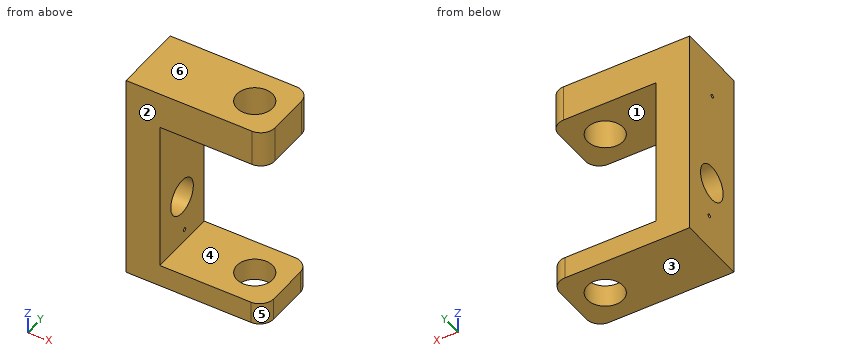
```python
from build123d import *

# Parameters (mm, degrees)
F0_W      = 50.8
F0_H      = 25.4
F1_DEPTH  = 76.2
F2_W      = 38.502306
F2_H      = 62.993251
F3_DEPTH  = 50.8
F5_R      = 6.477
F6_DEPTH  = 25.4
F7_W      = 25.4
F7_H      = 8.050508
F8_DEPTH  = 38.1
F4_R      = 6.477
F9_DEPTH  = 101.6
F10_R     = 5.08
F11_R     = 0.652616
F12_DEPTH = 25.4


with BuildPart() as f1:
    # F0 (on Top) → F1 (new body)
    with BuildSketch(Plane.XY):
        with Locations((-25.4, 12.7)):
            Rectangle(F0_W, F0_H)
    extrude(amount=F1_DEPTH)

    # F2 (on face) → F3 (cut)
    with BuildSketch(Plane.XZ):
        with Locations((-19.251153, 31.496625)):
            Rectangle(F2_W, F2_H)
    extrude(amount=-F3_DEPTH, mode=Mode.SUBTRACT)

    # F5 (on face) → F6 (cut)
    with BuildSketch(Plane(origin=(-50.8, 0, 0), x_dir=(0, -1, 0), z_dir=(-1, 0, 0))):
        with Locations((-12.7, 26.55393)):
            Circle(F5_R)
    extrude(amount=-F6_DEPTH, mode=Mode.SUBTRACT)

    # F7 (on face) → F8 (join)
    with BuildSketch(Plane.YZ.offset(-38.502306)):
        with Locations((12.7, 4.025254)):
            Rectangle(F7_W, F7_H)
    extrude(amount=F8_DEPTH)

    # F4 (on face) → F9 (cut)
    with BuildSketch(Plane.XY.offset(76.2)):
        with Locations((-12.11443, 12.7)):
            Circle(F4_R)
    extrude(amount=-F9_DEPTH, mode=Mode.SUBTRACT)

    # F10
    f10_edges = [f1.edges().sort_by_distance(p)[0] for p in [
        (0, 0, 69.596625),
        (-0.402306, 0, 4.025254),
        (-0.402306, 25.4, 4.025254),
        (0, 25.4, 69.596625),
    ]]
    fillet(f10_edges, radius=F10_R)

    # F11 (on face) → F12 (cut)
    with BuildSketch(Plane(origin=(-50.8, 0, 0), x_dir=(0, -1, 0), z_dir=(-1, 0, 0))):
        with Locations((-12.464834, 61.265279)):
            Circle(F11_R)
        with Locations((-14.175368, 12.515864)):
            Circle(F11_R)
    extrude(amount=-F12_DEPTH, mode=Mode.SUBTRACT)


solid = f1.part
```
Geometry check sheet. Reference: the model listing, model coordinates, mm. Face numbers are marked on the shaded views. A direction names the side the tool comes from. Give positions to 0.01 mm unless a question says otherwise; leave off trailing zeros. Loops run counter-clockwise (first coordinate to the right, second up) from the corner with the lowest first, then second, coordinate; pieces in that order, holes last. Notation, with made-up numbers: M -19.75,77 L 4.25,77 A15 cw 4.25,91 Z; hole C 20.25,-38 d5. An arc over 180 degrees is marked long. Write item = value, one per line.
(1) Sectioned sample at D-D, the plane z = 6.5. Record the cut outline in (x, y).
Answer below:
outline = M -50.8,0 L -5.48,0 A5.08 ccw -0.4,5.08 L -0.4,20.32 A5.08 ccw -5.48,25.4 L -50.8,25.4 Z; hole C -12.11,12.7 d12.95
(2) Release check for a two-part mould opening along Z. For the marked faces 3, 4, 5 and 6 record: released by +Z, released by -Z, zero draft, split by the parting line, or undercut.
Answer below:
face_3 = released by -Z
face_4 = undercut
face_5 = zero draft
face_6 = released by +Z
(3) Sectioned sample at C-C, the plane y = 10.5. Record the cut outline in (x, z).
Answer below:
outline = M -50.8,0 L -18.21,0 L -18.21,8.05 L -38.5,8.05 L -38.5,20.46 L -50.8,20.46 Z; M -50.8,32.65 L -38.5,32.65 L -38.5,62.99 L -18.21,62.99 L -18.21,76.2 L -50.8,76.2 Z; M -6.02,0 L -0.4,0 L -0.4,8.05 L -6.02,8.05 Z; M -6.02,62.99 L 0,62.99 L 0,76.2 L -6.02,76.2 Z
(4) Gauge pin test, flat ends, axial feed: pin 1 Ø10 at (y, z) = (17, 23.5) entering from +X; pin 2 Ø4 at (y, z) = (11.5, 3.5) entering from +X. Record the tip position at first contact, or that the pin passes through.
Answer below:
pin_1 = -38.5
pin_2 = -0.4
(5) Tool access check on the marked faces 1 and 2. Record the directions out of +Z, -Z, +X, -X, +Y, -Y that give a thin tool (end or side, any length) a straight path to the whole face; none if there is none.
Answer below:
face_1 = +X, +Y, -Y
face_2 = +Z, -Z, +X, -X, -Y
(6) Sectioned sample at A-A, the plane x = -28.5. Record the cut outline in (y, z).
Answer below:
outline = M 0,0 L 25.4,0 L 25.4,8.05 L 0,8.05 Z; M 0,62.99 L 25.4,62.99 L 25.4,76.2 L 0,76.2 Z
(7) Sectioned sample at B-B, the plane z = 70.5. Record the cut outline in (x, y).
Answer below:
outline = M -50.8,0 L -5.08,0 A5.08 ccw 0,5.08 L 0,20.32 A5.08 ccw -5.08,25.4 L -50.8,25.4 Z; hole C -12.11,12.7 d12.95
(8) Material ranges on line 1 (Z direction, x = -17.5, y = 5.5); line 2 (Z direction, x = -41.75, y = 12.7); line 3 (X direction, y = 2, z = 24), recorded low to high. Write a range as [from, to].
Answer below:
line_1 = [0, 8.05], [62.99, 76.2]
line_2 = [0, 20.08], [33.03, 60.66], [61.87, 76.2]
line_3 = [-50.8, -38.5]
